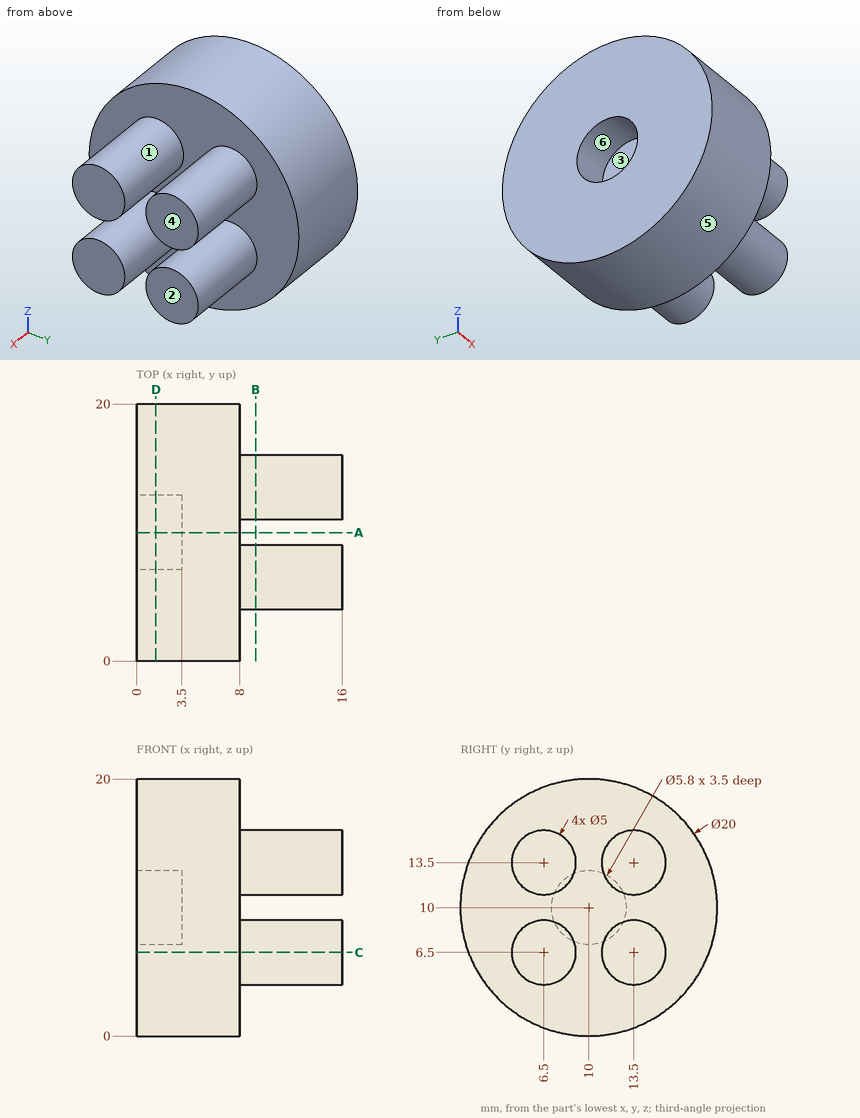
Can you work these out from the drawing? Everything is in mm from the part's minimum corner. A direction names the side the tool comes from. Give positions to 0.01 mm unless a question says otherwise; leave off trailing zeros. Order: outer loops, then holes, each group sorted by start corner. A loop starts at its lowest first (then second) coordinate and runs counter-clockwise, first axis right, second up.
Item 1: For the marked faces 1, 2 and 3, which set-ups out of +Z, -Z, +X, -X, +Y, -Y let a thin tool reach every point of the face, with its end or its side?
Item 2: I need wall thicknesses on line 1 (Y direction, x = 2.15, z = 10); line 2 (X direction, y = 16, z = 4.25); line 3 (Y direction, x = 10.75, z = 13.75). Which ranges of each line are inside material? Lowest first, please.
Item 3: If we section it at B-B, the plane x = 9.25: Write out the boundary of the cut face in (y, z).
Item 4: If we section it at A-A, the plane y = 10: Write out the boundary of the cut face in (x, z).
Item 5: I'm going to push flat-ended pins straight in: pin 1 (4 mm diameter, centred on x = 14, z = 11, fed in from -Y); pin 2 (1 mm diameter, centred on x = 10, y = 14, fed in from +Z); pin 3 (4 mm diameter, centred on x = 10.5, z = 14.5, fed in from -Y). Where does each tip first touch, or does it pass through?
Item 6: If we section it at D-D, the plane x = 1.5: Write out the boundary of the cut face in (y, z), plus the area to 3 significant figures.
Item 7: If we section it at C-C, the plane z = 6.5: Write out the boundary of the cut face in (x, y).
Item 8: If we mould it in two halves opening along Z, with no side actions, what happens to the marked faces 4, 5 and 6? For each: pulls with the +Z half, pulls with the -Z half, needs draft (parallel to the pull), parting line crosses it, or undercut.
Values:
1. face 1: +X
1. face 2: +Z, -Z, +X, +Y, -Y
1. face 3: -X
2. line 1: y = 0 to 7.1, 12.9 to 20
2. line 2: x = 0 to 8
2. line 3: y = 4.01 to 8.99, 11.01 to 15.99
3. outline: circle Ø5 at (6.5, 6.5); circle Ø5 at (6.5, 13.5); circle Ø5 at (13.5, 6.5); circle Ø5 at (13.5, 13.5)
4. outline: (0, 0) - (8, 0) - (8, 20) - (0, 20) - (0, 12.9) - (3.5, 12.9) - (3.5, 7.1) - (0, 7.1) - close
5. pin 1: stops at y = 4.05
5. pin 2: stops at z = 16
5. pin 3: stops at y = 4
6. outline: circle Ø20 at (10, 10); hole circle Ø5.8 at (10, 10)
6. area: 288 mm2
7. outline: (0, 0.63) - (8, 0.63) - (8, 4) - (16, 4) - (16, 9) - (8, 9) - (8, 11) - (16, 11) - (16, 16) - (8, 16) - (8, 19.37) - (0, 19.37) - close
8. face 4: needs draft
8. face 5: parting line crosses it
8. face 6: undercut
